Autodesk Inventor part; units mm, degrees
ref_plane "YZ Plane" through (0, 0, 0) normal (1, 0, 0) x (0, 1, 0)
ref_plane "XZ Plane" through (0, 0, 0) normal (0, 1, 0) x (-1, 0, 0)
ref_plane "XY Plane" through (0, 0, 0) normal (0, 0, 1) x (1, 0, 0)
sketch "スケッチ1" plane through (0, 0, 0) normal (0, 1, 0) x (-1, 0, 0)
  circle A0 centre (0, 0) radius 7
  dimension "d0" = 14
extrude "押し出し1" add sketch "スケッチ1" along normal blind 4
sketch "スケッチ2" plane through (0, 4, 0) normal (0, 1, 0) x (1, 0, 0)
  circle A0 centre (0, 0) radius 2.5
  dimension "d3" = 5
extrude "押し出し2" add sketch "スケッチ2" along normal blind 10
thread "ねじ1"
sketch "スケッチ3" plane through (0, 0, 0) normal (0, -1, 0) x (1, 0, 0)
  line L0 (10, 1) -> (-10, 1)
  line L1 (-10, 1) -> (-10, -1)
  line L2 (-10, -1) -> (10, -1)
  line L3 (10, -1) -> (10, 1)
  point P0 (0, 0)
  point P1 (0, 1)
  dimension "d8" = 20
  dimension "d9" = 2
  dimension "d10" = 1
  dimension "d11" = 10
extrude "押し出し3" cut sketch "スケッチ3" against normal blind 1.5
properties part number "camera_mount" material "アルミニウム 6061"
The model under review builds one solid part; all positions refer to its coordinate system, in mm. A direction names the side the tool comes from. Coordinates: 2 decimals unless noted, no trailing zeros. Loops run counter-clockwise (first coordinate to the right, second up) from the corner with the lowest first, then second, coordinate; pieces in that order, holes last. Notation, with made-up numbers: M 54,15.25 L 104,15.25 A17 ccw 104,19.25 Z; hole C 58.25,42.25 d7. An arc over 180 degrees is marked long. Put each result on its own line as item: value. Start each with the question number.
Q1. Add section B-B (x = 0). Write out the cut boundary in (y, z).
Q2. For faces 5 (the cylindrical face through (-0.54, 8.93, -2.44)), 6 (the flat face through (0, 0, -3)), 7 (the flat face through (0, 1, 1)), list the 3-axis set-ups (+Z, -Z, +X, -X, +Y, -Y) from which the entire face can be reached by the end or side of a thin tool; tool diameter is ignored.
Q3. The part is to be moulded in two halves that separate along Z. For faces 1 (the cylindrical face through (-6.677, 1.972, -2.103)), 2 (the flat face through (0, 14, 0)), 3 (the flat face through (0, 1.5, 0)), 4 (the flat face through (0, 1, -1)), say which applies: +Z half, -Z half, draft (parallel to the pull), parting line (faces both ways), or undercut.
Q4. Wall thickness on line 1 (Y direction, x = -1.5, z = -3.75); line 2 (X direction, y = 0.5, z = 3); line 3 (Z direction, x = -1.25, y = 13.25): over which ranges is each line inside the solid? List them lowest first.
Q5. Add section A-A (z = 0). Write out the cut boundary in (x, y).
Q6. Clearance check with flat-ended pins moving along their axes: pin 1 (1.6 mm diameter, centred on x = 2.5, y = 0.5, fed in from +Z); pin 2 (6 mm diameter, centred on x = -5.5, z = -5.5, fed in from +Y); pin 3 (3 mm diameter, centred on x = 3, y = 2.5, fed in from -Z). State where each tip first meets the part, or that it passes through.
Q7. Add section C-C (y = 10.5). Write out the cut boundary in (x, z).
Q8. Add section D-D (z = 1.5). Write out the cut boundary in (x, y), and give its area (3 significant figures).
Answers:
1. outline: M 0,-7 L 4,-7 L 4,-2.5 L 14,-2.5 L 14,2.5 L 4,2.5 L 4,7 L 0,7 L 0,1 L 1.5,1 L 1.5,-1 L 0,-1 Z
2. face 5: +Y
2. face 6: +Z, -Z, +X, -X, -Y
2. face 7: +X, -X, -Y
3. face 1: parting line
3. face 2: draft
3. face 3: undercut
3. face 4: undercut
4. line 1: y = 0 to 4
4. line 2: x = -6.32 to 6.32
4. line 3: z = -2.17 to 2.17
5. outline: M -7,1.5 L 7,1.5 L 7,4 L 2.5,4 L 2.5,14 L -2.5,14 L -2.5,4 L -7,4 Z
6. pin 1: stops at z = 6.79
6. pin 2: stops at y = 4
6. pin 3: stops at z = -6.84
7. outline: C 0,0 d5
8. outline: M -6.84,0 L 6.84,0 L 6.84,4 L 2,4 L 2,14 L -2,14 L -2,4 L -6.84,4 Z
8. area: 94.7 mm^2
